```python
from build123d import *

# Parameters (mm, degrees)
F0_W      = 134.9061876535
F0_H      = 66.3261953741
F1_DEPTH  = 50.8
F3_DEPTH  = 66.3271953741
F4_W      = 84.8675490558
F4_H      = 17.0645080507
F5_DEPTH  = 12.7
F7_DEPTH  = 12.7
F8_R      = 5.8831218442
F9_DEPTH  = 86.5717253991
F10_R     = 5.86386151
F10_R_2   = 6.47563258
F10_R_3   = 6.6609419445
F11_DEPTH = 86.5717253991
F13_DEPTH = 5.08


with BuildPart() as f1:
    # F0 (on Front) → F1 (new body)
    with BuildSketch(Plane.XZ):
        with Locations((2.2538006306, 3.86366155)):
            Rectangle(F0_W, F0_H)
    extrude(amount=F1_DEPTH)

    # F2 (on face) → F3 (cut, through all)
    with BuildSketch(Plane(origin=(0, 0, -29.2994361371), x_dir=(1, 0, 0), z_dir=(0, 0, -1))):
        Polygon((69.7068944573, 50.8), (19.6682558596, 50.8), (69.7068944573, 21.7111355625), align=None)
    extrude(amount=-F3_DEPTH, mode=Mode.SUBTRACT)

    # F4 (on face) → F5 (cut)
    with BuildSketch(Plane.XZ.offset(50.8)):
        with Locations((-22.7655186683, 8.5322540253)):
            Rectangle(F4_W, F4_H)
    extrude(amount=-F5_DEPTH, mode=Mode.SUBTRACT)

    # F6 (on face) → F7 (cut)
    with BuildSketch(Plane(origin=(27.0401800955, -46.5144936243, 0), x_dir=(0.864532465, 0.5025769761, 0), z_dir=(0.5025769761, -0.864532465, 0))):
        Polygon((-8.527064667, 17.0645080507), (-8.527064667, 0), (10.6996493414, 0), (10.6996493414, 17.1985588968), (-8.527064667, 17.1985588968), align=None)
    extrude(amount=-F7_DEPTH, mode=Mode.SUBTRACT)

    # F8 (on face) → F9 (cut, through all)
    with BuildSketch(Plane(origin=(27.0401800955, -46.5144936243, 0), x_dir=(0.864532465, 0.5025769761, 0), z_dir=(0.5025769761, -0.864532465, 0))):
        with Locations((8.8778939098, -14.6497180685)):
            Circle(F8_R)
    extrude(amount=-F9_DEPTH, mode=Mode.SUBTRACT)

    # F10 (on face) → F11 (cut, through all)
    with BuildSketch(Plane(origin=(27.0401800955, -46.5144936243, 0), x_dir=(0.864532465, 0.5025769761, 0), z_dir=(0.5025769761, -0.864532465, 0))):
        with Locations((33.0762192607, -15.5928293243)):
            Circle(F10_R)
        with Locations((17.0135609806, 27.9336217791)):
            Circle(F10_R_2)
        with Locations((38.3210889995, 28.7759676576)):
            Circle(F10_R_3)
    extrude(amount=-F11_DEPTH, mode=Mode.SUBTRACT)

    # F12 (on face) → F13 (cut)
    with BuildSketch(Plane(origin=(0, 0, -29.2994361371), x_dir=(1, 0, 0), z_dir=(0, 0, -1))):
        Polygon((69.7068944573, 21.7111355625), (19.6682558596, 50.8), (19.6682558596, 0), (69.7068944573, 0), align=None)
    extrude(amount=-F13_DEPTH, mode=Mode.SUBTRACT)


solid = f1.part
```
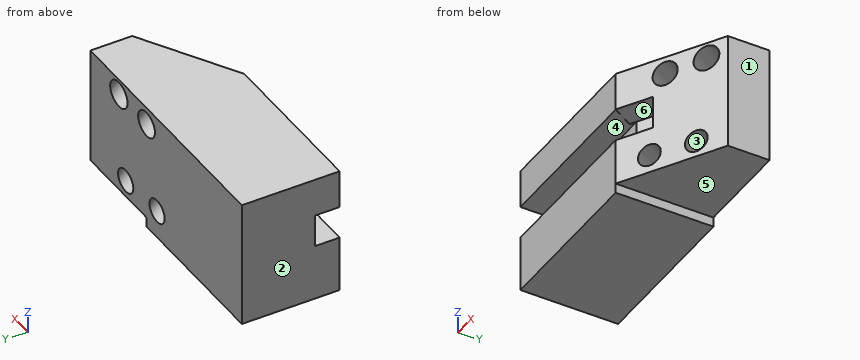
The listing builds one solid part. Answer for the finished solid, in the listing's coordinates (mm). Face numbers are marked on the shaded views. A direction names the side the tool comes from. Round coordinates to 2 decimals unless told otherwise and drop trailing zeros. Loops run counter-clockwise (first coordinate to the right, second up) from the corner with the lowest first, then second, coordinate; pieces in that order, holes last.
Q1. Find the intervals of material crossed by line 1 (X direction, y = -25, z = -15.5); line 2 (Z direction, x = -2, y = -46.5); line 3 (Z direction, x = 43, y = -8), in increasing order.
Q2. Section B-B, the plane z = 4 is taken. Determine the outline of the cut face in (x, y).
Q3. Section C-C, the plane x = -8 is taken. Determine the outline of the cut face in (y, z).
Q4. Section A-A, the plane z = 26.5 is taken. Determine the outline of the cut face in (x, y), then the cut area to 3 significant figures.
Q5. Which of the six approach directions +Z, -Z, +X, -X, +Y, -Y give full straight-line access (tool end or side, diameter ignored) to the marked faces 4, 5 and 6?
Q6. Given pin 1 Ø1.5 at (y, z) = (-36, -28) entering from +X; pin 2 Ø6 at (x, z) = (48, 29) entering from +Y; pin 3 Ø25 at (x, y) = (39.5, -27) entering from -Z, each flat-ended and moving along its own axis, determine where each tip first touches the part or whether it passes through.
Q7. Section D-D, the plane y = -5.5 is taken. Count the separate pieces of the cut face and the enclosed holes in it, then the cut area to 3 significant figures.
Q8. For a pull along X with two mould halves and no side action, classify the marked faces 1, 2 and 3 as released by +X, released by -X, zero draft, split by the parting line, or undercut.
Completed:
1. line 1: x = -65.2 to 18.07, 31.54 to 46.01, 59.57 to 64.05
1. line 2: z = -29.3 to 0, 17.06 to 37.03
1. line 3: z = -24.22 to -21.46, -9.73 to 24.57, 32.98 to 37.03
2. outline: (-65.2, -38.1) - (16.25, -38.1) - (29.91, -30.16) - (36.29, -41.14) - (69.71, -21.71) - (69.71, 0) - (-65.2, 0) - close
3. outline: (-50.8, -29.3) - (0, -29.3) - (0, 37.03) - (-50.8, 37.03) - (-50.8, 17.06) - (-38.1, 17.06) - (-38.1, 0) - (-50.8, 0) - close
4. outline: (-65.2, -50.8) - (19.67, -50.8) - (36.29, -41.14) - (12.38, 0) - (-65.2, 0) - close; (26.98, 0) - (47.21, -34.79) - (54.76, -30.4) - (37.08, 0) - close; (51.57, 0) - (65.58, -24.11) - (69.71, -21.71) - (69.71, 0) - close
4. area: 5,180 mm2
5. face 4: -X, -Y
5. face 5: -Z, +X, +Y, -Y
5. face 6: none
6. pin 1: stops at x = 19.67
6. pin 2: stops at y = -14.4
6. pin 3: stops at z = -24.22
7. separate pieces: 1
7. enclosed holes: 4
7. area: 8,130 mm2
8. face 1: released by +X
8. face 2: released by -X
8. face 3: undercut
